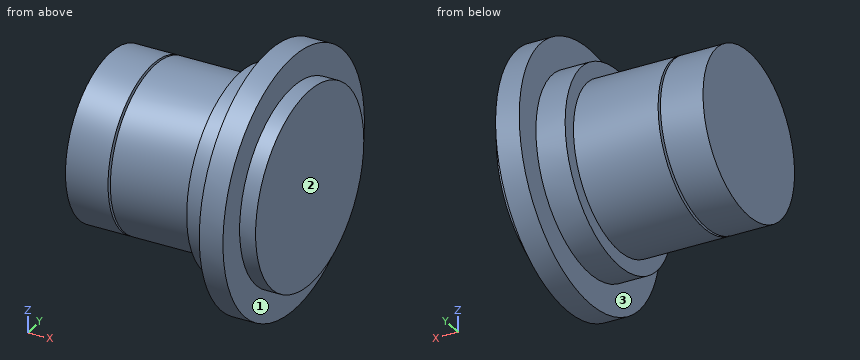
```python
from build123d import *

# Parameters (mm, degrees)
SKICA3_R                 = 38.468571429
SKICA3_R_2               = 6.2
ODEBRAT_VYSUNUT_M1_DEPTH = 1.1


with BuildPart() as part:
    # Skica1 → Rotovat1 (revolve)
    with BuildSketch(Plane.XY):
        Polygon((0, 0), (93.257142857, 0), (93.257142857, 45.462857143), (85.744761905, 45.462857143), (85.744761905, 59.451428571), (74.605714286, 59.451428571), (74.605714286, 45.462857143), (60.876190476, 45.462857143), (60.876190476, 38.468571429), (0, 38.468571429), align=None)
    revolve(axis=Axis((0, 0, 0), (-1, 0, 0)))

    # Skica3 → Odebrat vysunutím1 (cut)
    with BuildSketch(Plane.ZY.offset(-20)):
        Circle(SKICA3_R)
        Circle(SKICA3_R_2, mode=Mode.SUBTRACT)
    extrude(amount=-ODEBRAT_VYSUNUT_M1_DEPTH, mode=Mode.SUBTRACT)


solid = part.part
```
Geometry check sheet. Reference: the model listing, model coordinates, mm. Face numbers are marked on the shaded views. A direction names the side the tool comes from. Give positions to 0.01 mm unless a question says otherwise; leave off trailing zeros. Loops run counter-clockwise (first coordinate to the right, second up) from the corner with the lowest first, then second, coordinate; pieces in that order, holes last. Notation, with made-up numbers: M -37,51 L -14,51 A22 ccw -14,69 Z; hole C 83.5,48.25 d6. An arc over 180 degrees is marked long. Write item = value, one per line. Start each with the question number.
1. Go/stop test with flat-tipped pins: P1, Ø1, axis at x = 19, y = 15, coming from the -Z side; P2, Ø2, axis at x = 29.5, y = -17, coming from the +Z side; P3, Ø8, axis at y = -21.5, z = 46, coming from the -X side. Record where each tip stops, or that it passes through.
2. Section check D-D, the plane z = 16. Enter the section's corners in (x, y), plus the area to 3 significant figures.
3. Thickness scan on probe 1 along X at (y, z) = (20, -25); probe 2 along X at (y, z) = (-38, 12.5); probe 3 along X at (y, z) = (-30.5, -49.5). Record the ranges inside material, lowest first.
4. Tool access check on the marked faces 1, 2 and 3. Record the directions out of +Z, -Z, +X, -X, +Y, -Y that give a thin tool (end or side, any length) a straight path to the whole face; none if there is none.
5. Section check B-B, the plane z = 0. Enter the section's corners in (x, y), plus the area to 3 significant figures.
6. Section check A-A, the plane y = -12. Enter the section's corners in (x, z).
Values follow:
q1.P1 = -35.63
q1.P2 = 34.98
q1.P3 = 74.61
q2.outline = M 0,-34.98 L 20,-34.98 L 20,34.98 L 0,34.98 Z; M 21.1,-34.98 L 60.88,-34.98 L 60.88,-42.55 L 74.61,-42.55 L 74.61,-57.26 L 85.74,-57.26 L 85.74,-42.55 L 93.26,-42.55 L 93.26,42.55 L 85.74,42.55 L 85.74,57.26 L 74.61,57.26 L 74.61,42.55 L 60.88,42.55 L 60.88,34.98 L 21.1,34.98 Z
q2.area = 7,270 mm^2
q3.probe_1 = 0 to 20, 21.1 to 93.26
q3.probe_2 = 60.88 to 93.26
q3.probe_3 = 74.61 to 85.74
q4.face_1 = +X
q4.face_2 = +Z, -Z, +X, +Y, -Y
q4.face_3 = -X
q5.outline = M 0,-38.47 L 20,-38.47 L 20,-6.2 L 21.1,-6.2 L 21.1,-38.47 L 60.88,-38.47 L 60.88,-45.46 L 74.61,-45.46 L 74.61,-59.45 L 85.74,-59.45 L 85.74,-45.46 L 93.26,-45.46 L 93.26,45.46 L 85.74,45.46 L 85.74,59.45 L 74.61,59.45 L 74.61,45.46 L 60.88,45.46 L 60.88,38.47 L 21.1,38.47 L 21.1,6.2 L 20,6.2 L 20,38.47 L 0,38.47 Z
q5.area = 7,870 mm^2
q6.outline = M 0,-36.55 L 20,-36.55 L 20,36.55 L 0,36.55 Z; M 21.1,-36.55 L 60.88,-36.55 L 60.88,-43.85 L 74.61,-43.85 L 74.61,-58.23 L 85.74,-58.23 L 85.74,-43.85 L 93.26,-43.85 L 93.26,43.85 L 85.74,43.85 L 85.74,58.23 L 74.61,58.23 L 74.61,43.85 L 60.88,43.85 L 60.88,36.55 L 21.1,36.55 Z
